Source: CAD feature listing. Evaluate the final solid. Frame: model axes, mm. Face numbers are marked on the shaded views. Give positions to 0.01 mm unless a question says otherwise; leave off trailing zeros. Write each loop counter-clockwise with the first axis right and the second up, starting at its lowest first coordinate (ties: lowest second). Pieces come first, ordered by that corner, then holes. Notation, with made-up numbers: (-27.5, 29.25) -> (9.5, 29.25) arc R15 ccw to (9.5, 51.25) -> close; hole circle Ø6 at (-4, 73). An arc over 180 degrees is marked (long way). Answer as a JSON object with one key per item and string values. Group by question number.
Item 1: Section query C-C on z = -5.5. Return the cut outline in (x, y), plus the area to 3 significant figures.
Item 2: Ray query, probe 1 along Y at (x, z) = (0, 5); probe 2 along X at (y, z) = (0.25, -9); probe 3 along X at (y, z) = (-1, -22). Return the intervals inside material, ascending. Write a range as from..to.
Item 3: Section query A-A on x = 0. Return the cut outline in (y, z).
Item 4: First-contact query: pin 1 Ø4 at (x, y) = (1, 1) entering from -Z; pin 2 Ø3 at (x, y) = (0, 0) entering from +Z; pin 3 Ø2 at (y, z) = (-4, -14.5) entering from -X; pin 4 Ø6 at (x, y) = (0, 0) entering from -Z. Flat tips, straight axial feed; report the tip coordinate or a pass-through.
Item 5: Section query D-D on z = 2. Return the cut outline in (x, y), plus the area to 3 significant figures.
Item 6: Section query B-B on z = -25. Return the cut outline in (x, y).
Item 7: Pull-direction query (X, two-part tool) for the marked faces 1 and 2; classes: pulls with the +X half, pulls with the -X half, needs draft (parallel to the pull), parting line crosses it, or undercut.
from build123d import *

# Parameters (mm, degrees)
EXTRUDE_THIN1_DEPTH = 6
SKETCH2_R           = 5.65
SKETCH2_R_2         = 2.65
BOSS_EXTRUDE1_DEPTH = 13
BOSS_EXTRUDE2_START = 30
SKETCH3_R           = 5.65
BOSS_EXTRUDE2_DEPTH = 30
CHAMFER1_SIZE       = 0.5
CHAMFER2_SIZE       = 0.5
SKETCH4_R           = 2.65
CUT_EXTRUDE1_DEPTH  = 9
CUT_EXTRUDE2_DEPTH  = 6
CHAMFER3_SIZE       = 0.5
SKETCH8_OUTSIDE_W   = 22.474
SKETCH8_OUTSIDE_H   = 22.474
SKETCH8_OUTSIDE_R   = 5
CUT_EXTRUDE5_DEPTH  = 44.736083501
CHAMFER4_SIZE       = 0.5


with BuildPart() as part:
    # Sketch1 → Extrude-Thin1 (new body)
    with BuildSketch(Plane.XY):
        with BuildLine():
            Line((-1.843908891, 3.15), (1.843908891, 3.15))
            ThreePointArc((1.843908891, 3.15), (0, -3.65), (-1.843908891, 3.15))
        make_face()
        with BuildLine():
            Line((-1.549193338, 2.15), (1.549193338, 2.15))
            ThreePointArc((1.549193338, 2.15), (0, -2.65), (-1.549193338, 2.15))
        make_face(mode=Mode.SUBTRACT)
    extrude(amount=EXTRUDE_THIN1_DEPTH)

    # Sketch2 → Boss-Extrude1 (add)
    with BuildSketch(Plane(origin=(0, 0, 0), x_dir=(-1, 0, 0), z_dir=(0, 0, -1))):
        Circle(SKETCH2_R)
        Circle(SKETCH2_R_2, mode=Mode.SUBTRACT)
    extrude(amount=-BOSS_EXTRUDE1_DEPTH)

    # Sketch3 → Boss-Extrude2 (add)
    with BuildSketch(Plane(origin=(0, 0, 0), x_dir=(-1, 0, 0), z_dir=(0, 0, -1)).offset(BOSS_EXTRUDE2_START)):
        Circle(SKETCH3_R)
    extrude(amount=-BOSS_EXTRUDE2_DEPTH)

    # Chamfer1
    # the kernel refuses this chamfer: 0.5 mm, written as the material it takes off along each edge
    with BuildSketch(Plane(origin=(0, 0, 13), x_dir=(-1, 0, 0), z_dir=(0, -1, 0))) as chamfer1_piece_1:
        Polygon((2.65 + CHAMFER1_SIZE, 0), (2.65, CHAMFER1_SIZE), (2.65, 0), align=None)
    revolve(axis=Axis((0, 0, 13), (0, 0, -1)), mode=Mode.SUBTRACT)

    # Chamfer2
    chamfer2_edges = [part.edges().sort_by_distance(p)[0] for p in [
        (5.65, 0, 13),
    ]]
    chamfer(chamfer2_edges, length=CHAMFER2_SIZE)

    # Sketch4 → Cut-Extrude1 (cut)
    with BuildSketch(Plane(origin=(0, 0, -30), x_dir=(-1, 0, 0), z_dir=(0, 0, -1))):
        Circle(SKETCH4_R)
    extrude(amount=-CUT_EXTRUDE1_DEPTH, mode=Mode.SUBTRACT)

    # Sketch5 → Cut-Extrude2 (cut)
    with BuildSketch(Plane(origin=(0, 0, -21), x_dir=(-1, 0, 0), z_dir=(0, 0, -1))):
        with BuildLine():
            Line((1.549193338, 2.15), (-1.549193338, 2.15))
            ThreePointArc((-1.549193338, 2.15), (-1.207712228, -2.358798672), (2.65, 0))
            ThreePointArc((2.65, 0), (2.358798672, 1.207712228), (1.549193338, 2.15))
        make_face()
    extrude(amount=-CUT_EXTRUDE2_DEPTH, mode=Mode.SUBTRACT)

    # Chamfer3
    chamfer3_edges = [part.edges().sort_by_distance(p)[0] for p in [
        (5.65, 0, -30),
        (2.65, 0, -30),
    ]]
    chamfer(chamfer3_edges, length=CHAMFER3_SIZE)

    # Sketch8 outside → Cut-Extrude5 (cut, through all)
    with BuildSketch(Plane.XY.offset(13)):
        Rectangle(SKETCH8_OUTSIDE_W, SKETCH8_OUTSIDE_H)
        Circle(SKETCH8_OUTSIDE_R, mode=Mode.SUBTRACT)
    extrude(amount=-CUT_EXTRUDE5_DEPTH, mode=Mode.SUBTRACT)

    # Chamfer4
    chamfer4_edges = [part.edges().sort_by_distance(p)[0] for p in [
        (-5, 0, -30),
        (-5, 0, 13),
    ]]
    chamfer(chamfer4_edges, length=CHAMFER4_SIZE)


solid = part.part
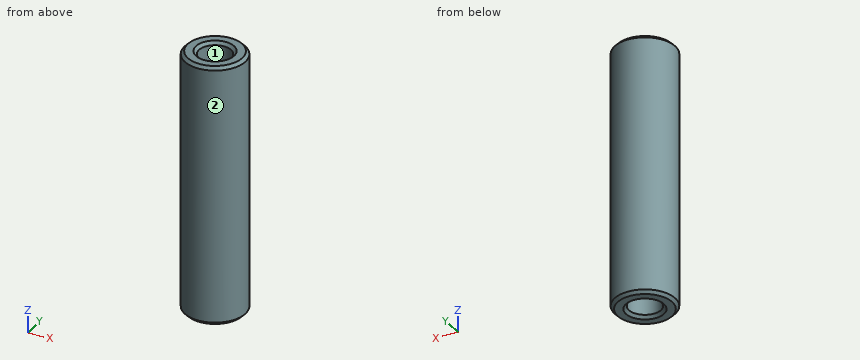
Worked answers:
{
 "1": {"outline": "circle Ø10 at (0, 0)", "area": "78.5 mm^2"},
 "2": {"probe 1": "-5..-2.65, 2.15..5", "probe 2": "-4.99..4.99", "probe 3": "-4.9..-2.45, 2.45..4.9"},
 "3": {"outline": "(-5, -29.5) -> (-4.5, -30) -> (-3.15, -30) -> (-2.65, -29.5) -> (-2.65, -15) -> (2.15, -15) -> (2.15, -21) -> (2.65, -21) -> (2.65, -29.5) -> (3.15, -30) -> (4.5, -30) -> (5, -29.5) -> (5, 12.5) -> (4.5, 13) -> (3.15, 13) -> (2.65, 12.5) -> (2.65, 6) -> (2.15, 6) -> (2.15, 0) -> (-2.65, 0) -> (-2.65, 12.5) -> (-3.15, 13) -> (-4.5, 13) -> (-5, 12.5) -> close"},
 "4": {"pin 1": "z = -30", "pin 2": "z = 0", "pin 3": "x = -4", "pin 4": "z = -29.85"},
 "5": {"outline": "circle Ø10 at (0, 0); hole (-1.55, 2.15) arc R2.65 ccw (long way) to (1.55, 2.15) -> close", "area": "57.5 mm^2"},
 "6": {"outline": "circle Ø10 at (0, 0); hole circle Ø5.3 at (0, 0)"},
 "7": {"face 1": "undercut", "face 2": "parting line crosses it"}
}
